```python
from build123d import *

# Parameters (mm, degrees)
SKETCH1_R           = 7.25
SKETCH1_R_2         = 3.25
BOSS_EXTRUDE1_DEPTH = 6
SKETCH2_R           = 6.5
SKETCH2_R_2         = 3.25
BOSS_EXTRUDE2_DEPTH = 5
CHAMFER1_SIZE       = 5
CHAMFER2_SIZE       = 2.5
CHAMFER2_SIZE2      = 9.330127019
FILLET1_R           = 40
CHAMFER3_SIZE       = 2.5
CHAMFER3_SIZE2      = 9.330127019
FILLET2_R           = 40


with BuildPart() as part:
    # Sketch1 → Boss-Extrude1 (new body)
    with BuildSketch(Plane.XY):
        with BuildLine():
            Line((-44.5, 0), (-44.5, -32))
            Line((-44.5, -32), (44.5, -32))
            Line((44.5, -32), (44.5, 0))
            ThreePointArc((44.5, 0), (29.5, 15), (14.5, 0))
            Line((14.5, 0), (-14.5, 0))
            ThreePointArc((-14.5, 0), (-29.5, 15), (-44.5, 0))
        make_face()
        with Locations((-29.5, 0)):
            Circle(SKETCH1_R, mode=Mode.SUBTRACT)
        with Locations(Location((29.5, 0, 0), (0, 0, 180))):
            Circle(SKETCH1_R, mode=Mode.SUBTRACT)
        with Locations((0, -17)):
            Circle(SKETCH1_R_2, mode=Mode.SUBTRACT)
    extrude(amount=BOSS_EXTRUDE1_DEPTH)

    # Sketch2 → Boss-Extrude2 (add)
    with BuildSketch(Plane.XY.offset(6)):
        with Locations(Location((0, -17, 0), (0, 0, 180))):
            Circle(SKETCH2_R)
        with Locations((0, -17)):
            Circle(SKETCH2_R_2, mode=Mode.SUBTRACT)
    extrude(amount=BOSS_EXTRUDE2_DEPTH)

    # Chamfer1
    chamfer1_edges = [part.edges().sort_by_distance(p)[0] for p in [
        (6.5, -17, 6),
    ]]
    chamfer(chamfer1_edges, length=CHAMFER1_SIZE - 0.0001)  # a hair under: the kernel refuses the full size

    # Chamfer2
    chamfer2_edges = [part.edges().sort_by_distance(p)[0] for p in [
        (-44.5, -32, 3),
    ]]
    chamfer2_side = [part.faces().sort_by_distance(p)[0] for p in [
        (0, -32, 3),
    ]]
    chamfer(chamfer2_edges, length=CHAMFER2_SIZE, length2=CHAMFER2_SIZE2, reference=chamfer2_side[0])

    # Fillet1
    fillet1_edges = [part.edges().sort_by_distance(p)[0] for p in [
        (-44.5, -22.669872981, 3),
    ]]
    fillet(fillet1_edges, radius=FILLET1_R)

    # Chamfer3
    chamfer3_edges = [part.edges().sort_by_distance(p)[0] for p in [
        (44.5, -32, 3),
    ]]
    chamfer3_side = [part.faces().sort_by_distance(p)[0] for p in [
        (1.25, -32, 3),
    ]]
    chamfer(chamfer3_edges, length=CHAMFER3_SIZE, length2=CHAMFER3_SIZE2, reference=chamfer3_side[0])

    # Fillet2
    fillet2_edges = [part.edges().sort_by_distance(p)[0] for p in [
        (44.5, -22.669872981, 3),
    ]]
    fillet(fillet2_edges, radius=FILLET2_R)


solid = part.part
```
The model under review builds one solid part; all positions refer to its coordinate system, in mm. A direction names the side the tool comes from. Round coordinates to 2 decimals unless told otherwise and drop trailing zeros. Write each loop counter-clockwise with the first axis right and the second up, starting at its lowest first coordinate (ties: lowest second). Pieces come first, ordered by that corner, then holes.
(1) Machinability: for faces 1 (the flat face through (44.5, -9, 3)), 2 (the flat face through (0, 0, 3)), which of the approach directions +Z, -Z, +X, -X, +Y, -Y give a long, thin tool a straight path to every point of the face, cutting with its end or side? Answer none if there is none.
(2) We need section C-C on y = -1. Give the boundary of the cut face in (x, z).
(3) Wall thickness on L1, parallel to X at y = -2.5, z = 5; L2, parallel to Y at x = -29.5, z = 3.3; L3, parallel to Z at x = -27.5, y = -13.5: over which ranges is each line inside the solid? List them lowest first.
(4) We need section D-D on y = 6. Give the boundary of the cut face in (x, z), and give its area (3 significant figures).
(5) Mouldability with a two-part tool opening along X and no side actions: class faces 3 (the cylindrical face through (44.148, -22.697, 3.042)), 4 (the flat face through (-1, -32, 3)), 5 (the cylindrical face through (29.83, 14.996, 2.958)) as +X half, -X half, draft (parallel to the pull), parting line (faces both ways), or undercut.
(6) We need section B-B on z = 2.25. Give the boundary of the cut face in (x, y).
(7) Insertion check: pin 1 (1.8 mm diameter, centred on x = 7, z = 4, fed in from +Y); pin 2 (3 mm diameter, centred on y = 5, z = 2, fed in from +X). Each pin has a flat end and moves straight along its axis. Give the tip position at first contact, or say it passes through.
Findings below:
1. face 1: +Z, -Z, +X, +Y, -Y
1. face 2: +Z, -Z, +Y
2. outline: (-44.5, 0) - (-36.68, 0) - (-36.68, 6) - (-44.5, 6) - close; (-22.32, 0) - (22.32, 0) - (22.32, 6) - (-22.32, 6) - close; (36.68, 0) - (44.5, 0) - (44.5, 6) - (36.68, 6) - close
3. L1: x = -44.5 to -36.31, -22.69 to 22.69, 36.31 to 44.5
3. L2: y = -32 to -7.25, 7.25 to 15
3. L3: z = 0 to 6
4. outline: (-43.25, 0) - (-33.57, 0) - (-33.57, 6) - (-43.25, 6) - close; (-25.43, 0) - (-15.75, 0) - (-15.75, 6) - (-25.43, 6) - close; (15.75, 0) - (25.43, 0) - (25.43, 6) - (15.75, 6) - close; (33.57, 0) - (43.25, 0) - (43.25, 6) - (33.57, 6) - close
4. area: 232 mm2
5. face 3: +X half
5. face 4: draft
5. face 5: undercut
6. outline: (-44.5, -17.4) arc R40 ccw to (-43.14, -27.76) - (-42, -32) - (42, -32) - (43.14, -27.76) arc R40 ccw to (44.5, -17.4) - (44.5, 0) arc R15 ccw to (14.5, 0) - (-14.5, 0) arc R15 ccw to (-44.5, 0) - close; hole circle Ø14.5 at (-29.5, 0); hole circle Ø6.5 at (0, -17); hole circle Ø14.5 at (29.5, 0)
7. pin 1: stops at y = 0
7. pin 2: stops at x = 44.09
